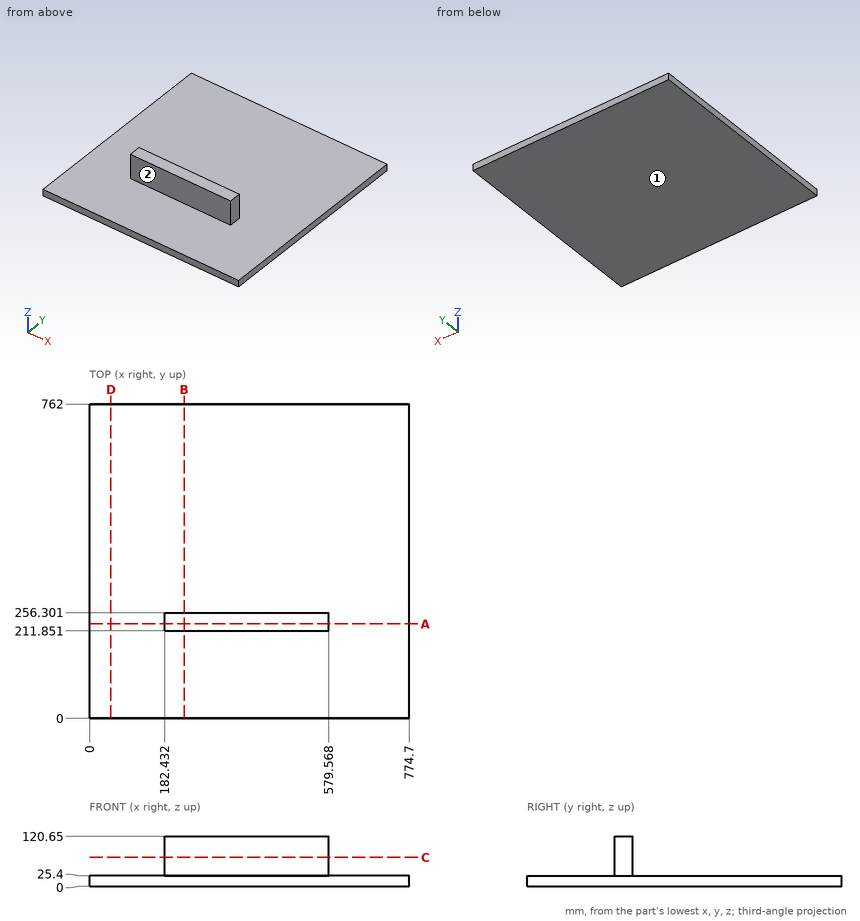
Geometry check sheet. Reference: drawing and pictorial views, mm from the part's lowest x, y, z. A direction names the side the tool comes from. Coordinates: 2 decimals unless noted, no trailing zeros. Loops run counter-clockwise (first coordinate to the right, second up) from the corner with the lowest first, then second, coordinate; pieces in that order, holes last. Notation, with made-up numbers: (45.25, -17.5) - (75.25, -17.5) arc R20 ccw to (75.25, -13.5) - close; hole circle Ø6 at (38, 11). An arc over 180 degrees is marked (long way). Return JSON: item names as keys, results as strings.
1. Tool access check on the marked faces 1 and 2. Record the directions out of +Z, -Z, +X, -X, +Y, -Y that give a thin tool (end or side, any length) a straight path to the whole face; none if there is none.
Established:
{"face 1": "-Z, +X, -X, +Y, -Y", "face 2": "+Z, +X, -X, -Y"}
2. Go/stop test with flat-tipped pins: pin 1 (12 mm diameter, centred on x = 612.5, y = 284.5, fed in from -Z); pin 2 (4 mm diameter, centred on x = 97, y = 235, fed in from +Z); pin 3 (22 mm diameter, centred on y = 245, z = 52, fed in from -X); pin 4 (22 mm diameter, centred on y = 227.5, z = 83.5, fed in from +X). Record where each tip stops, or that it passes through.
Established:
{"pin 1": "stops at z = 0", "pin 2": "stops at z = 25.4", "pin 3": "stops at x = 182.43", "pin 4": "stops at x = 579.57"}
3. Thickness scan on L1, parallel to Y at x = 269, z = 115; L2, parallel to Z at x = 487, y = 87. Record the ranges inside material, lowest first.
Established:
{"L1": "y = 211.85 to 256.3", "L2": "z = 0 to 25.4"}
4. Section check C-C, the plane z = 70. Record the boundary of the cut face in (x, y).
Established:
{"outline": "(182.43, 211.85) - (579.57, 211.85) - (579.57, 256.3) - (182.43, 256.3) - close"}
5. Section check D-D, the plane x = 52. Record the boundary of the cut face in (y, z).
Established:
{"outline": "(0, 0) - (762, 0) - (762, 25.4) - (0, 25.4) - close"}
6. Section check A-A, the plane y = 229. Record the boundary of the cut face in (x, z).
Established:
{"outline": "(0, 0) - (774.7, 0) - (774.7, 25.4) - (579.57, 25.4) - (579.57, 120.65) - (182.43, 120.65) - (182.43, 25.4) - (0, 25.4) - close"}
7. Section check B-B, the plane x = 229.5. Record the boundary of the cut face in (y, z), then the cut area to 3 significant figures.
Established:
{"outline": "(0, 0) - (762, 0) - (762, 25.4) - (256.3, 25.4) - (256.3, 120.65) - (211.85, 120.65) - (211.85, 25.4) - (0, 25.4) - close", "area": "23,600 mm2"}
